Model file for the job. Use its own axes, mm. A direction names the side the tool comes from. Give positions to 0.01 mm unless a question says otherwise; leave off trailing zeros. Loops run counter-clockwise (first coordinate to the right, second up) from the corner with the lowest first, then second, coordinate; pieces in that order, holes last. Notation, with made-up numbers: (37, 82) - (80, 82) arc R17 ccw to (80, 108) - close; hole circle Ø9 at (75.25, -18.75). An arc over 180 degrees is marked (long way). Use a Markdown table: item, result.
from build123d import *

# Parameters (mm, degrees)
CHAMFER1_SIZE      = 0.3
CUT_EXTRUDE1_DEPTH = 1


with BuildPart() as part:
    # Sketch2 → Revolve1 (revolve)
    with BuildSketch(Plane.XY):
        with BuildLine():
            Line((0, 0), (39.15, 0))
            Line((39.15, 0), (39.15, 1.5))
            Line((39.15, 1.5), (1.65, 1.5))
            Line((1.65, 1.5), (1.65, 2.85))
            Line((1.65, 2.85), (1.3, 2.85))
            ThreePointArc((1.3, 2.85), (0.549895392, 2.228823502), (0, 1.425))
            Line((0, 1.425), (0, 0))
        make_face()
    revolve(axis=Axis((0, 0, 0), (1, 0, 0)))

    # Chamfer1
    chamfer1_edges = [part.edges().sort_by_distance(p)[0] for p in [
        (39.15, -1.5, 0),
    ]]
    chamfer(chamfer1_edges, length=CHAMFER1_SIZE)

    # Sketch3 → Cut-Extrude1 (cut)
    with BuildSketch(Plane.ZY):
        Polygon((0.576043408, 1.000753379), (-0.578656145, 0.999244915), (-1.154699553, -0.001508464), (-0.576043408, -1.000753379), (0.578656145, -0.999244915), (1.154699553, 0.001508464), align=None)
    extrude(amount=-CUT_EXTRUDE1_DEPTH, mode=Mode.SUBTRACT)


solid = part.part
(1) 3-axis set-ups, long thin cutter, end or side, ignore diameter. For faces 4 (the flat face through (0.49, -0.51, 0.86)), 5 (the cylindrical face through (19.99, -1.5, 0.07)), 6 (the flat face through (39.15, 0, 0)): which of +Z, -Z, +X, -X, +Y, -Y reach the whole face in a straight line?
Computed:
| item | result |
|---|---|
| face 4 | -X |
| face 5 | +X |
| face 6 | +Z, -Z, +X, +Y, -Y |
(2) Pin check, flat tips, straight feed: P1, Ø2, axis at x = 10, y = -1, coming from the +Z side; P2, Ø2, axis at x = 35, z = -1, coming from the -Y side; P3, Ø1.5, axis at x = 23, z = 0, coming from the +Y side. Stop position of each tip, or through.
Computed:
| item | result |
|---|---|
| P1 | z = 1.5 |
| P2 | y = -1.5 |
| P3 | y = 1.5 |
(3) Slice it at A-A, the plane x = 4. Write the cut outline in (y, z).
Computed:
| item | result |
|---|---|
| outline | circle Ø3 at (0, 0) |
(4) Mould opens along Z. For faces 1 (the flat face through (0.49, 0.51, -0.86)), 2 (the flat face through (1.65, -1.2, -1.2)), 3 (the cylindrical face through (1.473, -2.262, -1.734)) say: pulls with the +Z half, pulls with the -Z half, needs draft (parallel to the pull), parting line crosses it, or undercut.
Computed:
| item | result |
|---|---|
| face 1 | undercut |
| face 2 | needs draft |
| face 3 | parting line crosses it |
(5) Drill centre lines: probe 1 along Z at (x, y) = (22, 0.05); probe 2 along X at (y, z) = (0.65, -2.15). Where is each one in solid material? Low to high. Write a range as [from, to].
Computed:
| item | result |
|---|---|
| probe 1 | [-1.5, 1.5] |
| probe 2 | [0.57, 1.65] |
